Input: part model. Units: mm. Frame: model coordinates. Face numbers are marked on the shaded views. A direction names the side the tool comes from. Coordinates: 2 decimals unless noted, no trailing zeros. Order: outer loops, then holes, each group sorted by start corner. A loop starts at its lowest first (then second) coordinate and runs counter-clockwise, first axis right, second up. Notation, with made-up numbers: (22, -34.5) - (52, -34.5) arc R20 ccw to (52, -25.5) - close; hole circle Ø6 at (86.25, 29). An arc over 180 degrees is marked (long way). One line per question, with ' | ' between items.
from build123d import *

# Parameters (mm, degrees)
SKETCH4_R           = 3.96875
SKETCH4_R_2         = 5.2959
SKETCH4_R_3         = 1.5
SKETCH4_R_4         = 3.175
BOSS_EXTRUDE2_DEPTH = 10.16
FILLET1_R           = 3.81


with BuildPart() as part:
    # Sketch4 → Boss-Extrude2 (new body)
    with BuildSketch(Plane(origin=(0, 0, 0), x_dir=(1, 0, 0), z_dir=(0, 1, 0))):
        with BuildLine():
            Line((54.2925, 31.75), (-12.3825, 31.75))
            Line((-12.3825, 31.75), (-7.863361559, -1.082336008))
            ThreePointArc((-7.863361559, -1.082336008), (-3.056289676, -7.325503373), (4.7625, -6.35))
            Line((4.7625, -6.35), (41.91, -6.35))
            ThreePointArc((41.91, -6.35), (45.967580476, -4.884520517), (48.152310263, -1.164501002))
            Line((48.152310263, -1.164501002), (54.2925, 31.75))
        make_face()
        Circle(SKETCH4_R, mode=Mode.SUBTRACT)
        with Locations((46.355, 22.86)):
            Circle(SKETCH4_R, mode=Mode.SUBTRACT)
        with Locations((-4.445, 22.86)):
            Circle(SKETCH4_R, mode=Mode.SUBTRACT)
        with Locations((16.764, 8.636)):
            Circle(SKETCH4_R_2, mode=Mode.SUBTRACT)
        with Locations((27.264, 8.636)):
            Circle(SKETCH4_R_3, mode=Mode.SUBTRACT)
        with Locations((6.264, 8.636)):
            Circle(SKETCH4_R_3, mode=Mode.SUBTRACT)
        with Locations((41.91, 0)):
            Circle(SKETCH4_R_4, mode=Mode.SUBTRACT)
        with BuildLine():
            Line((34.925, 29.21), (6.985, 29.21))
            ThreePointArc((6.985, 29.21), (5.188948776, 28.466051224), (4.445, 26.67))
            Line((4.445, 26.67), (4.445, 19.1135))
            ThreePointArc((4.445, 19.1135), (5.188948776, 17.317448776), (6.985, 16.5735))
            Line((6.985, 16.5735), (34.925, 16.5735))
            ThreePointArc((34.925, 16.5735), (36.721051224, 17.317448776), (37.465, 19.1135))
            Line((37.465, 19.1135), (37.465, 26.67))
            ThreePointArc((37.465, 26.67), (36.721051224, 28.466051224), (34.925, 29.21))
        make_face(mode=Mode.SUBTRACT)
        with BuildLine():
            Line((46.58698696, 4.295147609), (48.631735848, 15.256028661))
            ThreePointArc((48.631735848, 15.256028661), (44.519378774, 15.137668683), (40.900146495, 17.093850549))
            Line((40.900146495, 17.093850549), (38.737442476, 5.500670755))
            ThreePointArc((38.737442476, 5.500670755), (42.873923491, 6.276412312), (46.58698696, 4.295147609))
        make_face(mode=Mode.SUBTRACT)
        with BuildLine():
            Line((36.83, -3.81), (6.963318623, -3.81))
            ThreePointArc((6.963318623, -3.81), (7.800370345, -1.469057088), (7.872207457, 1.016))
            Line((7.872207457, 1.016), (35.641806959, 1.016))
            ThreePointArc((35.641806959, 1.016), (35.744131016, -1.518077625), (36.83, -3.81))
        make_face(mode=Mode.SUBTRACT)
        with BuildLine():
            Line((-6.14066773, 5.029523445), (-7.591897143, 15.572960504))
            ThreePointArc((-7.591897143, 15.572960504), (-3.525796009, 14.975903966), (0.293891225, 16.492361803))
            Line((0.293891225, 16.492361803), (1.490851578, 7.796234208))
            ThreePointArc((1.490851578, 7.796234208), (-2.705340953, 7.462240721), (-6.14066773, 5.029523445))
        make_face(mode=Mode.SUBTRACT)
        with BuildLine():
            Line((35.921478098, 7.718896983), (36.959282513, 13.2820499))
            ThreePointArc((36.959282513, 13.2820499), (36.823503538, 13.804258048), (36.335051487, 14.0335))
            Line((36.335051487, 14.0335), (27.003423807, 14.0335))
            ThreePointArc((27.003423807, 14.0335), (26.395931126, 13.583371961), (26.649696678, 12.871146117))
            Line((26.649696678, 12.871146117), (34.943519943, 7.307993201))
            ThreePointArc((34.943519943, 7.307993201), (35.543221805, 7.249922938), (35.921478098, 7.718896983))
        make_face(mode=Mode.SUBTRACT)
    extrude(amount=BOSS_EXTRUDE2_DEPTH)

    # Fillet1
    fillet1_edges = [part.edges().sort_by_distance(p)[0] for p in [
        (-12.3825, 5.08, -31.75),
        (54.2925, 5.08, -31.75),
    ]]
    fillet(fillet1_edges, radius=FILLET1_R)


solid = part.part
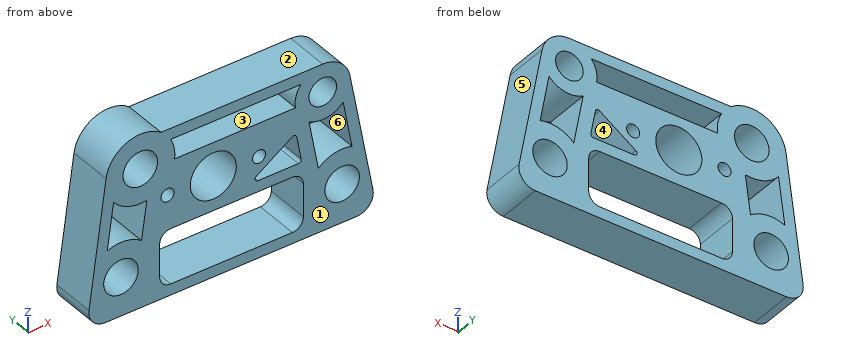
Item 1: Section D-D on y = 6. Count the separate pieces of the cut face and the enclosed holes in it, and give its area (3 significant figures).
Data:
separate pieces: 1 | enclosed holes: 12 | area: 1,280 mm^2
Item 2: Section A-A on x = 25. Return the cut outline in (y, z).
Data:
outline: (0, -31.75) - (10.16, -31.75) - (10.16, -29.21) - (0, -29.21) - close; (0, -16.57) - (10.16, -16.57) - (10.16, -1.02) - (0, -1.02) - close; (0, 3.81) - (10.16, 3.81) - (10.16, 6.35) - (0, 6.35) - close
Item 3: Access query for the marked faces 5 and 6. Directions: +Z, -Z, +X, -X, +Y, -Y. A direction counts if a zero-diameter tool reaches every point of the face in a straight line with its end or side. Return the directions, or none.
Data:
face 5: +Z, +X, +Y, -Y | face 6: +Y, -Y
Item 4: Section C-C on x = 17. Return the cut outline in (y, z).
Data:
outline: (0, -31.75) - (10.16, -31.75) - (10.16, -29.21) - (0, -29.21) - close; (0, -16.57) - (10.16, -16.57) - (10.16, -13.93) - (0, -13.93) - close; (0, -3.35) - (10.16, -3.35) - (10.16, -1.02) - (0, -1.02) - close; (0, 3.81) - (10.16, 3.81) - (10.16, 6.35) - (0, 6.35) - close
Item 5: Ray query, line 1 (Z direction, x = 9, y = 4.25); line 2 (Z direction, x = 16.5, y = 3.75); line 3 (X direction, y = 1.75, z = -26.5) (3 decimals). Return the intervals inside material, ascending.
Data:
line 1: -31.75 to -29.21, -16.57 to -1.02, 3.81 to 6.35 | line 2: -31.75 to -29.21, -16.57 to -13.93, -3.35 to -1.02, 3.81 to 6.35 | line 3: -11.66 to -6.027, -2.863 to 4.445, 37.465 to 44.773, 47.937 to 53.313
Item 6: Draft query along Z for the marked faces 1, 2, 3 and 4. Return one class per face: released by +Z, released by -Z, zero draft, split by the parting line, or undercut.
Data:
face 1: zero draft | face 2: released by +Z | face 3: undercut | face 4: undercut
Item 7: Contact query for flat-ended pins moving along their axis: P1, Ø5, axis at y = 6.5, z = -8.5, coming from the -X side; P2, Ø5, axis at x = 28.5, y = 4, coming from the +Z side; P3, Ø1, axis at y = 7.5, z = -25.5, coming from the -X side; P4, Ø9.5, axis at x = 16.764, z = -8.636, coming from the +Y side. Output: stop coordinate, or through.
Data:
P1: x = -9.53 | P2: z = 6.35 | P3: x = -11.59 | P4: through
Item 8: Section B-B on z = 0. Return the cut outline in (x, y) (1 decimal), and give its area (3 significant figures).
Data:
outline: (-8, 0) - (-4, 0) - (-4, 10.2) - (-8, 10.2) - close; (4, 0) - (7.9, 0) - (7.9, 10.2) - (4, 10.2) - close; (35.6, 0) - (38.7, 0) - (38.7, 10.2) - (35.6, 10.2) - close; (45.1, 0) - (48.4, 0) - (48.4, 10.2) - (45.1, 10.2) - close | area: 147 mm^2
